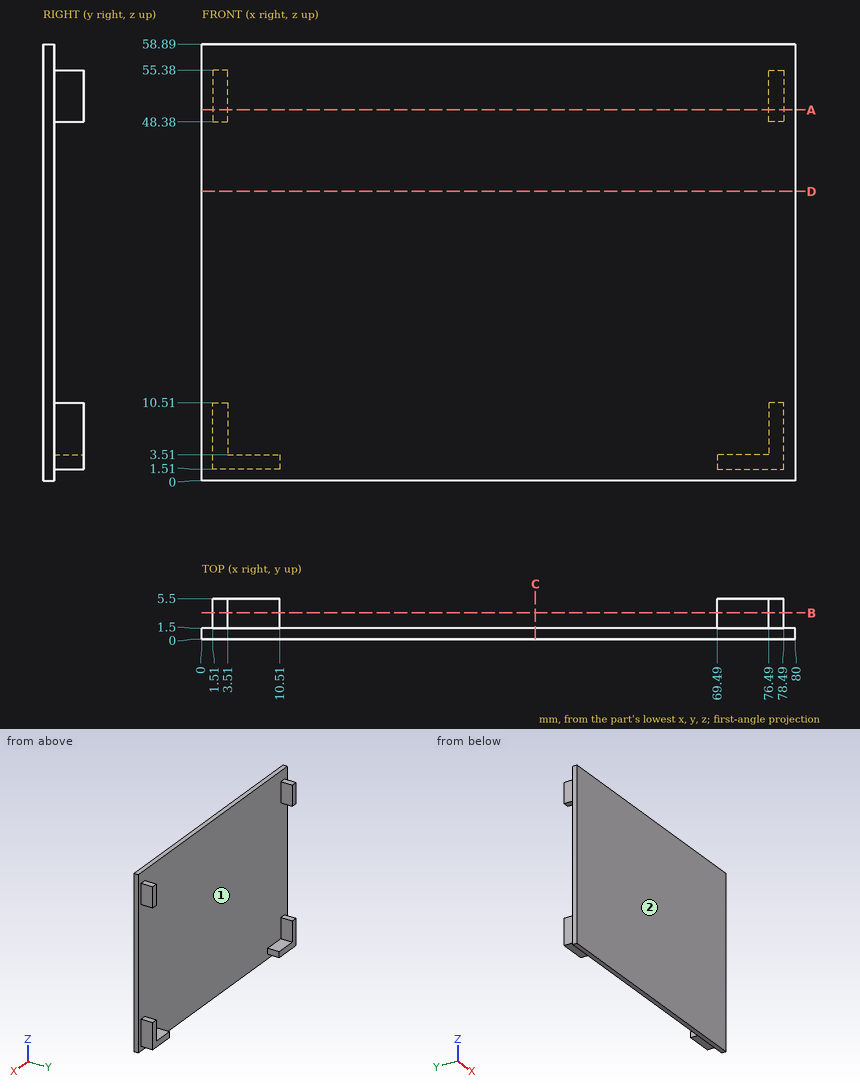
Input: dimensioned drawing with shaded views. Units: mm. Origin: part minimum x, y, z. Round coordinates to 2 decimals unless told otherwise and drop trailing zeros. Write each loop counter-clockwise with the first axis right and the second up, starting at its lowest first coordinate (ties: lowest second). Pieces come first, ordered by that corner, then holes. Notation, with made-up numbers: (54, -5) - (75, -5) arc R16 ccw to (75, 26) - close; hole circle Ø8 at (-12, 69). An arc over 180 degrees is marked (long way). Write item = value, one per line.
(1) Section query B-B on y = 3.6. Output: boundary loops of the cut face in (x, z), then the cut area to 3 significant figures.
Geometry check:
outline = (1.51, 1.51) - (10.51, 1.51) - (10.51, 3.51) - (3.51, 3.51) - (3.51, 10.51) - (1.51, 10.51) - close; (1.51, 48.38) - (3.51, 48.38) - (3.51, 55.38) - (1.51, 55.38) - close; (69.49, 1.51) - (78.49, 1.51) - (78.49, 10.51) - (76.49, 10.51) - (76.49, 3.51) - (69.49, 3.51) - close; (76.49, 48.38) - (78.49, 48.38) - (78.49, 55.38) - (76.49, 55.38) - close
area = 92.0 mm^2
(2) Pull-direction query (X, two-part tool) for the marked faces 1 and 2; classes: +X half, -X half, draft (parallel to the pull), parting line (faces both ways), or undercut.
Geometry check:
face_1 = undercut
face_2 = draft
(3) Material intervals for probe 1 along X at (y, z) = (3.9, 7.5); probe 2 along Y at (x, z) = (68, 48); probe 3 along Z at (x, y) = (5, 4.45), sorted ascending.
Geometry check:
probe_1 = 1.51 to 3.51, 76.49 to 78.49
probe_2 = 0 to 1.5
probe_3 = 1.51 to 3.51
(4) Section query D-D on z = 39. Output: boundary loops of the cut face in (x, y).
Geometry check:
outline = (0, 0) - (80, 0) - (80, 1.5) - (0, 1.5) - close
(5) Section query A-A on z = 50. Output: boundary loops of the cut face in (x, y), then the cut area to 3 significant figures.
Geometry check:
outline = (0, 0) - (80, 0) - (80, 1.5) - (78.49, 1.5) - (78.49, 5.5) - (76.49, 5.5) - (76.49, 1.5) - (3.51, 1.5) - (3.51, 5.5) - (1.51, 5.5) - (1.51, 1.5) - (0, 1.5) - close
area = 136 mm^2
(6) Section query C-C on x = 45. Output: boundary loops of the cut face in (y, z), then the cut area to 3 significant figures.
Geometry check:
outline = (0, 0) - (1.5, 0) - (1.5, 58.89) - (0, 58.89) - close
area = 88.3 mm^2
(7) Contact query for flat-ended pins moving along their axis: pin 1 Ø8 at (x, z) = (19.5, 17.5) entering from +Y; pin 2 Ø2 at (y, z) = (3, 3) entering from +X; pin 3 Ø1.2 at (x, y) = (8.5, 4) entering from +Z. Output: stop coordinate, or through.
Geometry check:
pin_1 = 1.5
pin_2 = 78.49
pin_3 = 3.51
